from build123d import *

# Parameters (mm, degrees)
SKETCH1_W               = 100
SKETCH1_H               = 70
BOSS_EXTRUDE1_DEPTH     = 20
SKETCH2_R               = 4
CUT_EXTRUDE1_DEPTH      = 21
CUT_EXTRUDE1_DEPTH_BACK = 1
SKETCH3_R               = 7.5
CUT_EXTRUDE2_DEPTH      = 15
SKETCH4_W               = 100
SKETCH4_H               = 1
CUT_EXTRUDE3_DEPTH      = 21
CUT_EXTRUDE3_DEPTH_BACK = 1


with BuildPart() as part:
    # Sketch1 → Boss-Extrude1 (new body)
    with BuildSketch(Plane.XY):
        Rectangle(SKETCH1_W, SKETCH1_H)
    extrude(amount=BOSS_EXTRUDE1_DEPTH)

    # Sketch2 → Cut-Extrude1 (cut, two sides)
    with BuildSketch(Plane.XY) as cut_extrude1_sk:
        with Locations((-41, 0)):
            Circle(SKETCH2_R)
        with Locations((41, 0)):
            Circle(SKETCH2_R)
    extrude(amount=CUT_EXTRUDE1_DEPTH, mode=Mode.SUBTRACT)
    extrude(cut_extrude1_sk.sketch, amount=-CUT_EXTRUDE1_DEPTH_BACK, mode=Mode.SUBTRACT)

    # Sketch3 → Cut-Extrude2 (cut)
    with BuildSketch(Plane.XY.offset(20)):
        Circle(SKETCH3_R)
    extrude(amount=-CUT_EXTRUDE2_DEPTH, mode=Mode.SUBTRACT)

    # Sketch4 → Cut-Extrude3 (cut, two sides)
    with BuildSketch(Plane.XY) as cut_extrude3_sk:
        with Locations((0, -34.5)):
            Rectangle(SKETCH4_W, SKETCH4_H)
    extrude(amount=CUT_EXTRUDE3_DEPTH, mode=Mode.SUBTRACT)
    extrude(cut_extrude3_sk.sketch, amount=-CUT_EXTRUDE3_DEPTH_BACK, mode=Mode.SUBTRACT)


solid = part.part
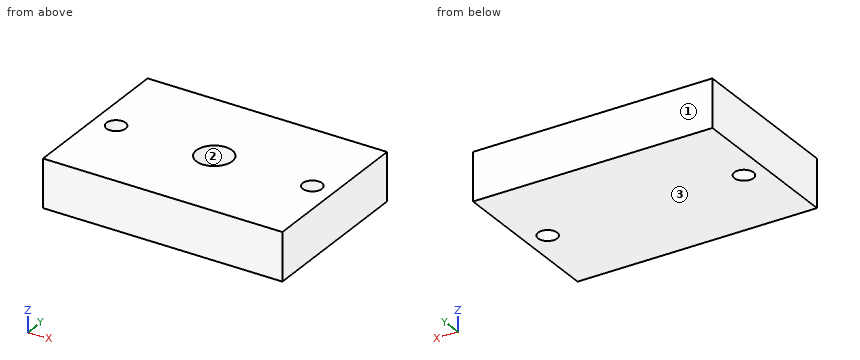
Read the model definition and answer for the solid it produces. Units are mm, in the model's axes. Face numbers are marked on the shaded views. Round coordinates to 2 decimals unless told otherwise and drop trailing zeros. Write each loop counter-clockwise with the first axis right and the second up, starting at its lowest first coordinate (ties: lowest second). Pieces come first, ordered by that corner, then holes.
1. The part is cut by section B-B, the plane z = 18.5. Determine the outline of the cut face in (x, y), then the cut area to 3 significant figures.
2. The part is cut by section C-C, the plane x = 41. Determine the outline of the cut face in (y, z).
3. Straight lines are drawn through the part: L1, parallel to Y at x = 41, z = 11.75; L2, parallel to Y at x = 0, z = 14.75; L3, parallel to Z at x = -1.5, y = -1. For each, find the intervals that lie inside material, in ascending order.
4. The part is cut by section D-D, the plane x = 0. Determine the outline of the cut face in (y, z), then the cut area to 4 significant figures.
5. Determine the mould class of the marked faces 1, 2 and 3 for opening direction Y: pulls with the +Y half, pulls with the -Y half, needs draft (parallel to the pull), parting line crosses it, or undercut.
6. The part is cut by section A-A, the plane y = 0. Determine the outline of the cut face in (x, z).
Values:
1. outline: (-50, -34) - (50, -34) - (50, 35) - (-50, 35) - close; hole circle Ø8 at (-41, 0); hole circle Ø15 at (0, 0); hole circle Ø8 at (41, 0)
1. area: 6,620 mm2
2. outline: (-34, 0) - (-4, 0) - (-4, 20) - (-34, 20) - close; (4, 0) - (35, 0) - (35, 20) - (4, 20) - close
3. L1: y = -34 to -4, 4 to 35
3. L2: y = -34 to -7.5, 7.5 to 35
3. L3: z = 0 to 5
4. outline: (-34, 0) - (35, 0) - (35, 20) - (7.5, 20) - (7.5, 5) - (-7.5, 5) - (-7.5, 20) - (-34, 20) - close
4. area: 1,155 mm2
5. face 1: pulls with the +Y half
5. face 2: undercut
5. face 3: needs draft
6. outline: (-50, 0) - (-45, 0) - (-45, 20) - (-50, 20) - close; (-37, 0) - (37, 0) - (37, 20) - (7.5, 20) - (7.5, 5) - (-7.5, 5) - (-7.5, 20) - (-37, 20) - close; (45, 0) - (50, 0) - (50, 20) - (45, 20) - close
